Read the model definition and answer for the solid it produces. Units are mm, in the model's axes. A direction names the side the tool comes from. Round coordinates to 2 decimals unless told otherwise and drop trailing zeros. Order: outer loops, then holes, each group sorted by start corner. A loop starts at its lowest first (then second) coordinate and runs counter-clockwise, first axis right, second up. Notation, with made-up numbers: (83, 17) - (130, 17) arc R25 cw to (130, 49) - close; hole circle Ø4 at (7, 8.5). An arc over 180 degrees is marked (long way). Answer as a JSON object with one key per item and string values. Group by question number.
Q1. A cutting plane is placed at C-C on y = -5.5. Determine the outline of the cut face in (x, z), and give its area (3 significant figures).
Q2. A cutting plane is placed at D-D on z = -148.5. Determine the outline of the cut face in (x, y).
Q3. Consider line 1 (Z direction, x = -71, y = 6); line 2 (X direction, y = -21, z = -159); line 3 (Z direction, x = -70.5, y = -21). Determine where each line is inside the solid, lowest interval first.
Q4. Given pin 1 Ø8 at (x, z) = (-8.5, -114) entering from -Y, flat-ended and moving along its own axis, determine where the tip first touches the part or whether it passes through.
Q5. The mould has two halves that part along X. Classify faces 4 (the flat face through (-101, -13, -165.1)), 5 (the flat face through (-146.05, 2, 2)), 6 (the flat face through (-140, -13, -101.6)): pulls with the +X half, pulls with the -X half, needs draft (parallel to the pull), parting line crosses it, or undercut.
Q6. A tool of negligible diameter and unlimited length cuts with its end or side. For faces 1 (the flat face through (-69.85, -13, -172)), 2 (the cylindrical face through (15.877, 6.439, -0.14)), 3 (the flat face through (133.35, -13, 134)), from which of +Z, -Z, +X, -X, +Y, -Y can it reach the whole face along a straight path? Write none if from no direction.
Q7. A cutting plane is placed at B-B on z = 0. Determine the outline of the cut face in (x, y) (3 decimals).
Q8. A cutting plane is placed at A-A on x = 29.5. Determine the outline of the cut face in (y, z), and give its area (3 significant figures).
```python
from build123d import *

# Parameters (mm, degrees)
SKETCH1_W           = 292.1
SKETCH1_H           = 355.6
SKETCH1_W_2         = 215.9
SKETCH1_H_2         = 279.4
BOSS_EXTRUDE1_DEPTH = 12.7
CUT_EXTRUDE1_DEPTH  = 13.7
BOSS_EXTRUDE2_DEPTH = 25.4


with BuildPart() as part:
    # Sketch1 → Boss-Extrude1 (new body)
    with BuildSketch(Plane(origin=(0, 0, 0), x_dir=(1, 0, 0), z_dir=(0, 1, 0))):
        Rectangle(SKETCH1_W, SKETCH1_H)
        Polygon((-69.85, 139.7), (69.85, 139.7), (69.85, 152.4), (120.65, 152.4), (120.65, 101.6), (107.95, 101.6), (107.95, -101.6), (120.65, -101.6), (120.65, -152.4), (69.85, -152.4), (69.85, -139.7), (-69.85, -139.7), (-69.85, -152.4), (-120.65, -152.4), (-120.65, -101.6), (-107.95, -101.6), (-107.95, 101.6), (-120.65, 101.6), (-120.65, 152.4), (-69.85, 152.4), align=None, mode=Mode.SUBTRACT)
        Polygon((-107.95, 139.7), (-69.85, 139.7), (-69.85, 152.4), (-120.65, 152.4), (-120.65, 101.6), (-107.95, 101.6), align=None)
        Polygon((-107.95, -139.7), (-107.95, -101.6), (-120.65, -101.6), (-120.65, -152.4), (-69.85, -152.4), (-69.85, -139.7), align=None)
        Rectangle(SKETCH1_W_2, SKETCH1_H_2)
        Polygon((120.65, -101.6), (107.95, -101.6), (107.95, -139.7), (69.85, -139.7), (69.85, -152.4), (120.65, -152.4), align=None)
        Polygon((69.85, 152.4), (69.85, 139.7), (107.95, 139.7), (107.95, 101.6), (120.65, 101.6), (120.65, 152.4), align=None)
    extrude(amount=BOSS_EXTRUDE1_DEPTH)

    # Sketch2 → Cut-Extrude1 (cut, through all)
    with BuildSketch(Plane(origin=(0, 12.7, 0), x_dir=(1, 0, 0), z_dir=(0, 1, 0))):
        with BuildLine():
            Line((-123.825, 6.35), (-22.225, 6.35))
            ThreePointArc((-22.225, 6.35), (-15.875, 0), (-22.225, -6.35))
            Line((-22.225, -6.35), (-123.825, -6.35))
            ThreePointArc((-123.825, -6.35), (-130.175, 0), (-123.825, 6.35))
        make_face()
        with BuildLine():
            Line((123.825, 6.35), (22.225, 6.35))
            ThreePointArc((22.225, 6.35), (15.875, 0), (22.225, -6.35))
            Line((22.225, -6.35), (123.825, -6.35))
            ThreePointArc((123.825, -6.35), (130.175, 0), (123.825, 6.35))
        make_face()
    extrude(amount=-CUT_EXTRUDE1_DEPTH, mode=Mode.SUBTRACT)

    # Sketch3 → Boss-Extrude2 (add)
    with BuildSketch(Plane.XZ):
        Polygon((-69.85, 177.8), (-146.05, 177.8), (-146.05, 101.6), (-133.35, 101.6), (-133.35, 165.1), (-69.85, 165.1), align=None)
        Polygon((146.05, 177.8), (69.85, 177.8), (69.85, 165.1), (133.35, 165.1), (133.35, 101.6), (146.05, 101.6), align=None)
        Polygon((146.05, -177.8), (146.05, -101.6), (133.35, -101.6), (133.35, -165.1), (69.85, -165.1), (69.85, -177.8), align=None)
        Polygon((-133.35, -101.6), (-146.05, -101.6), (-146.05, -177.8), (-69.85, -177.8), (-69.85, -165.1), (-133.35, -165.1), align=None)
    extrude(amount=BOSS_EXTRUDE2_DEPTH)


solid = part.part
```
Result set:
{
 "1": {"outline": "(-146.05, -177.8) - (-69.85, -177.8) - (-69.85, -165.1) - (-133.35, -165.1) - (-133.35, -101.6) - (-146.05, -101.6) - close; (-146.05, 101.6) - (-133.35, 101.6) - (-133.35, 165.1) - (-69.85, 165.1) - (-69.85, 177.8) - (-146.05, 177.8) - close; (69.85, -177.8) - (146.05, -177.8) - (146.05, -101.6) - (133.35, -101.6) - (133.35, -165.1) - (69.85, -165.1) - close; (69.85, 165.1) - (133.35, 165.1) - (133.35, 101.6) - (146.05, 101.6) - (146.05, 177.8) - (69.85, 177.8) - close", "area": "7,100 mm²"},
 "2": {"outline": "(-146.05, -25.4) - (-133.35, -25.4) - (-133.35, 0) - (133.35, 0) - (133.35, -25.4) - (146.05, -25.4) - (146.05, 12.7) - (-146.05, 12.7) - close"},
 "3": {"line 1": "z = -177.8 to -6.35, 6.35 to 177.8", "line 2": "x = -146.05 to -133.35, 133.35 to 146.05", "line 3": "z = -177.8 to -165.1, 165.1 to 177.8"},
 "4": {"pin 1": "stops at y = 0"},
 "5": {"face 4": "undercut", "face 5": "pulls with the -X half", "face 6": "needs draft"},
 "6": {"face 1": "+Z, -Z, -Y", "face 2": "+Y, -Y", "face 3": "-Y"},
 "7": {"outline": "(-146.05, 0) - (-130.175, 0) - (-130.175, 12.7) - (-146.05, 12.7) - close; (-15.875, 0) - (15.875, 0) - (15.875, 12.7) - (-15.875, 12.7) - close; (130.175, 0) - (146.05, 0) - (146.05, 12.7) - (130.175, 12.7) - close"},
 "8": {"outline": "(0, -177.8) - (12.7, -177.8) - (12.7, -6.35) - (0, -6.35) - close; (0, 6.35) - (12.7, 6.35) - (12.7, 177.8) - (0, 177.8) - close", "area": "4,350 mm²"}
}
